Check sheet for the modelled part. Datum: model origin and axes. Units: mm. Face numbers are marked on the shaded views. Round coordinates to 2 decimals unless told otherwise and drop trailing zeros. Write each loop counter-clockwise with the first axis right and the second up, starting at its lowest first coordinate (ties: lowest second). Pieces come first, ordered by that corner, then holes. Notation, with made-up numbers: (2, 44) -> (25, 44) arc R30 ccw to (25, 67) -> close; hole circle Ø1 at (-24, 26). An arc over 180 degrees is marked (long way). One line per item, written item: value.
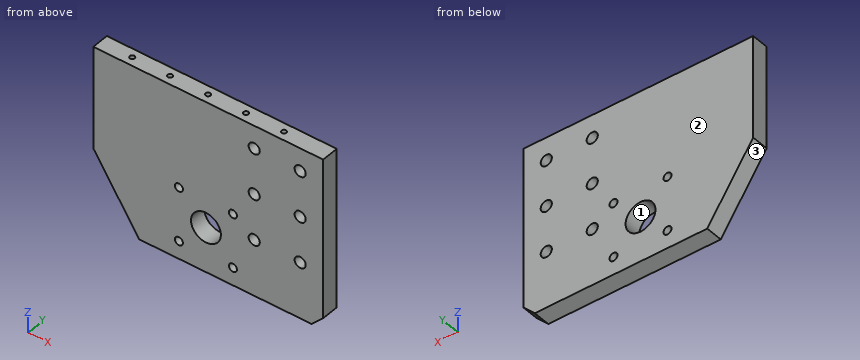
from build123d import *

# Parameters (mm, degrees)
F0_R      = 13
F1_DEPTH  = 15
F3_D      = 9.7
F5_D      = 7
F6_DEPTH  = 4
F7_DEPTH  = 55
F9_DEPTH  = 25
F11_D     = 4.2
F11_DEPTH = 15
F11_TIP   = 1.2618073


with BuildPart() as f1:
    # F0 (on Front) → F1 (new body)
    with BuildSketch(Plane.XZ):
        Polygon((73.4297142857, -49.4285714286), (73.4297142857, 89.5714285714), (-48.5702857143, 89.5714285714), (-67.5702857143, 89.5714285714), (-67.5702857143, 29.5714285714), (-67.5702857143, -59.4285714286), (63.4297142857, -59.4285714286), align=None)
        with Locations((-28.5702857143, -20.4285714286)):
            Circle(F0_R, mode=Mode.SUBTRACT)
    extrude(amount=F1_DEPTH)

    # F3 (through all)
    with Locations(Plane(origin=(0, 0, 0), x_dir=(-1, 0, 0), z_dir=(0, 1, 0))):
        with Locations((-53.4297142857, -10.4285714286), (-53.4297142857, 29.5714285714), (-53.4297142857, 69.5714285714), (-13.4297142857, 69.5714285714), (-13.4297142857, 29.5714285714), (-13.4297142857, -10.4285714286)):
            Hole(F3_D / 2)

    # F5 (through all)
    with Locations(Plane.XZ.offset(15)):
        with Locations((-52.0702857143, 3.0714285714), (-52.0702857143, -43.9285714286), (-5.0702857143, -43.9285714286), (-5.0702857143, 3.0714285714)):
            Hole(F5_D / 2)

    # F6 (add): a face of the model
    f6_faces = [f1.faces().sort_by_distance(p)[0] for p in [
        (-67.5702857143, -7.5, 15.0714285714),
    ]]
    extrude(f6_faces, amount=F6_DEPTH)

    # F7 (add): a face of the model
    f7_faces = [f1.faces().sort_by_distance(p)[0] for p in [
        (-71.5702857143, -7.5, 15.0714285714),
    ]]
    extrude(f7_faces, amount=F7_DEPTH)

    # F8 (on face) → F9 (cut)
    with BuildSketch(Plane(origin=(0, 0, 0), x_dir=(-1, 0, 0), z_dir=(0, 1, 0))):
        Polygon((126.5702857143, -59.4285714286), (126.5702857143, 0.5714285714), (86.5702857143, -59.4285714286), align=None)
    extrude(amount=-F9_DEPTH, mode=Mode.SUBTRACT)

    # F11
    with Locations(Plane.XY.offset(89.5714285714)):
        with Locations((-98.5702857143, -7.5), (-65.5702857143, -7.5), (-32.5702857143, -7.5), (0.4297142857, -7.5), (33.4297142857, -7.5)):
            Hole(F11_D / 2, depth=F11_DEPTH)
            with Locations((0, 0, -(F11_DEPTH + F11_TIP / 2))):  # 118° drill point
                Cone(0, F11_D / 2, F11_TIP, mode=Mode.SUBTRACT)


solid = f1.part
Item 1: Sectioned sample at B-B on y = -12.25. Count the separate pieces of the cut face and the enclosed holes in it, and give its area (3 significant figures).
Answer:
separate pieces: 1
enclosed holes: 11
area: 27,400 mm^2
Item 2: Depth check by flat-ended pin: P1, Ø9, axis at x = -52.07, z = -43.93, coming from the +Y side; P2, Ø4, axis at x = -98.57, y = -7.5, coming from the +Z side. Enter the tip coordinate at first touch or a pass-through.
Answer:
P1: stops at y = 0
P2: stops at z = 74.51
Item 3: Sectioned sample at C-C on x = -110.5. Enter the section's corners in (y, z).
Answer:
outline: (-15, -23.53) -> (0, -23.53) -> (0, 89.57) -> (-15, 89.57) -> close
Item 4: Mould release check, pull along Z, two halves, no side actions. Record for the marked faces 1, 2 and 3: pulls with the +Z half, pulls with the -Z half, needs draft (parallel to the pull), parting line crosses it, or undercut.
Answer:
face 1: undercut
face 2: needs draft
face 3: pulls with the -Z half
Item 5: Thickness scan on line 1 (X direction, y = -7.5, z = 86.5); line 2 (Z direction, x = -8, y = -7.75); line 3 (X direction, y = -9, z = 78). Record the ranges inside material, lowest first.
Answer:
line 1: x = -126.57 to -100.67, -96.47 to -67.67, -63.47 to -34.67, -30.47 to -1.67, 2.53 to 31.33, 35.53 to 73.43
line 2: z = -59.43 to -45.84, -42.01 to 1.16, 4.99 to 89.57
line 3: x = -126.57 to -100.04, -97.1 to -67.04, -64.1 to -34.04, -31.1 to -1.04, 1.9 to 31.96, 34.9 to 73.43
Item 6: Sectioned sample at A-A on x = -19. Enter the section's corners in (y, z), and give its area (3 significant figures).
Answer:
outline: (-15, -59.43) -> (0, -59.43) -> (0, -29.23) -> (-15, -29.23) -> close; (-15, -11.63) -> (0, -11.63) -> (0, 89.57) -> (-15, 89.57) -> close
area: 1,970 mm^2
